from build123d import *

# Parameters (mm, degrees)
FRONT_SKETCH_R      = 1.905
BOSS_EXTRUDE1_DEPTH = 50.8
CUT_EXTRUDE1_DEPTH  = 45.72
CUT_EXTRUDE2_DEPTH  = 274.638700861
CUT_EXTRUDE3_DEPTH  = 18.03621965
SKETCH6_W           = 6.524310643
SKETCH6_H           = 22.300846009
SKETCH6_R           = 1.524
SKETCH6_W_2         = 6.962786951
BOSS_EXTRUDE2_DEPTH = 10.16


with BuildPart() as part:
    # front_sketch → Boss-Extrude1 (new body)
    with BuildSketch(Plane(origin=(0, 0, 0), x_dir=(1, 0, 0), z_dir=(0, 1, 0))):
        with BuildLine():
            Line((-94.961375831, 124.478458264), (-121.345326632, 110.234521439))
            ThreePointArc((-121.345326632, 110.234521439), (-122.32001306, 109.300728329), (-122.678671172, 107.99944144))
            Line((-122.678671172, 107.99944144), (-122.678671172, 48.810796684))
            Line((-122.678671172, 48.810796684), (-140.250849959, 48.810796684))
            Line((-140.250849959, 48.810796684), (-140.250849959, -56.645199257))
            Line((-140.250849959, -56.645199257), (-119.167015715, -56.645199257))
            Line((-119.167015715, -56.645199257), (-119.167015715, -126.112255785))
            Line((-119.167015715, -126.112255785), (-95.601645083, -136.460242597))
            Line((-95.601645083, -136.460242597), (-95.601645083, -142.810242597))
            Line((-95.601645083, -142.810242597), (-105.798207048, -142.810242597))
            ThreePointArc((-105.798207048, -142.810242597), (-119.167015715, -139.007347839), (-128.532661201, -128.737404395))
            ThreePointArc((-128.532661201, -128.737404395), (-157.286213724, -5.861503432), (-127.918775374, 116.869125935))
            ThreePointArc((-127.918775374, 116.869125935), (-118.556014486, 127.058910858), (-105.241228699, 130.828458264))
            Line((-105.241228699, 130.828458264), (-94.961375831, 130.828458264))
            Line((-94.961375831, 130.828458264), (-94.961375831, 124.478458264))
        make_face()
        with Locations((-131.296368682, 71.963600743)):
            Circle(FRONT_SKETCH_R, mode=Mode.SUBTRACT)
        with Locations((-131.296368682, -86.786399257)):
            Circle(FRONT_SKETCH_R, mode=Mode.SUBTRACT)
    extrude(amount=BOSS_EXTRUDE1_DEPTH)

    # Sketch1 → Cut-Extrude1 (cut)
    with BuildSketch(Plane(origin=(0, 50.8, 0), x_dir=(1, 0, 0), z_dir=(0, 1, 0))):
        Polygon((-122.678671172, 48.810796684), (-122.678671172, 107.99944144), (-138.833286115, 78.405119062), (-140.250849959, 48.810796684), align=None)
        Polygon((-119.167015715, -56.645199257), (-140.250849959, -56.645199257), (-139.542068037, -96.192486205), (-119.167015715, -126.112255785), align=None)
    extrude(amount=-CUT_EXTRUDE1_DEPTH, mode=Mode.SUBTRACT)

    # Sketch3 → Cut-Extrude2 (cut, through all)
    with BuildSketch(Plane.XY.offset(142.810242597)):
        Polygon((-94.961375831, 50.8), (-157.287069608, 21.270817167), (-157.287069608, 50.8), align=None)
    extrude(amount=-CUT_EXTRUDE2_DEPTH, mode=Mode.SUBTRACT)

    # Sketch4 → Cut-Extrude3 (cut, through all)
    with BuildSketch(Plane(origin=(-140.250849959, 0, 0), x_dir=(0, 0, -1), z_dir=(1, 0, 0))):
        Polygon((-24.404629664, 24.144542412), (20.256333242, 24.144542412), (20.256333242, 5.094542412), (20.256333242, 1.843696403), (-24.404629664, 1.843696403), (-24.404629664, 5.094542412), align=None)
    extrude(amount=-CUT_EXTRUDE3_DEPTH, mode=Mode.SUBTRACT)

    # Sketch6 → Boss-Extrude2 (add)
    with BuildSketch(Plane(origin=(-140.250849959, 0, 0), x_dir=(0, 0, -1), z_dir=(1, 0, 0))):
        with Locations((-21.142474343, 12.994119407)):
            Rectangle(SKETCH6_W, SKETCH6_H)
        with Locations((-20.530013168, 12.991512488)):
            Circle(SKETCH6_R, mode=Mode.SUBTRACT)
        with Locations((16.774939767, 12.994119407)):
            Rectangle(SKETCH6_W_2, SKETCH6_H)
        with Locations((16.553986832, 12.991512488)):
            Circle(SKETCH6_R, mode=Mode.SUBTRACT)
    extrude(amount=-BOSS_EXTRUDE2_DEPTH)


solid = part.part
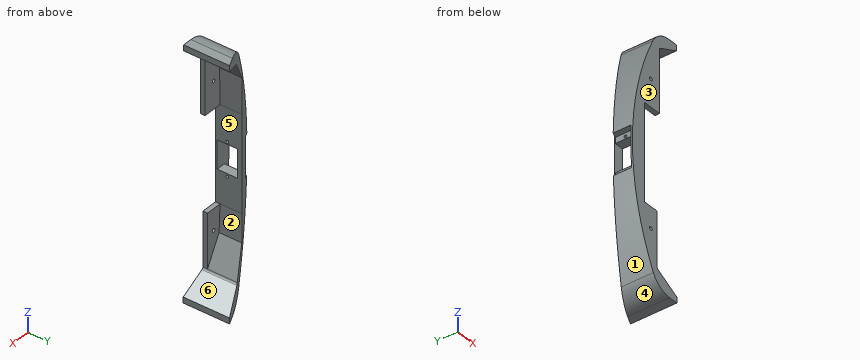
Geometry check sheet. Reference: the model listing, model coordinates, mm. Face numbers are marked on the shaded views. A direction names the side the tool comes from. Give positions to 0.01 mm unless a question says otherwise; leave off trailing zeros. Write each loop counter-clockwise with the first axis right and the second up, starting at its lowest first coordinate (ties: lowest second). Pieces come first, ordered by that corner, then holes.
1) Go/stop test with flat-tipped pins: pin 1 Ø3.5 at (x, z) = (-131.3, 86.79) entering from -Y; pin 2 Ø3.5 at (y, z) = (11.5, -16) entering from -X; pin 3 Ø9 at (x, z) = (-133, -89.5) entering from +Y; pin 4 Ø1.5 at (y, z) = (3, -71.5) entering from +X. Record where each tip stops, or that it passes through.
Values follow:
pin 1: passes through
pin 2: stops at x = -150.41
pin 3: stops at y = 33.88
pin 4: stops at x = -122.68
2) Set-up check for the marked faces 1 and 2: record each of +Z, -Z, +X, -X, +Y, -Y from which the full face is reachable in a straight line by a thin tool's end or side.
Values follow:
face 1: -X, +Y, -Y
face 2: +X, +Y
3) Release check for a two-part mould opening along Z. For the marked faces 3, 4, 5 and 6 record: released by +Z, released by -Z, zero draft, split by the parting line, or undercut.
Values follow:
face 3: zero draft
face 4: released by -Z
face 5: undercut
face 6: undercut
4) Cross-section at A-A (y = 8). Record the boundary of the cut face in (x, z), plus the area to 3 significant figures.
Values follow:
outline: (-156.7, 24.4) - (-150.41, 24.4) - (-150.41, 17.88) - (-140.25, 17.88) - (-140.25, 56.65) - (-139.54, 96.19) - (-119.17, 126.11) - (-95.6, 136.46) - (-95.6, 142.81) - (-105.8, 142.81) arc R25.4 ccw to (-128.53, 128.74) arc R274 ccw to start; (-155.97, -20.26) arc R274 ccw to (-127.92, -116.87) arc R25.4 ccw to (-105.24, -130.83) - (-94.96, -130.83) - (-94.96, -124.48) - (-121.35, -110.23) arc R2.54 cw to (-122.68, -108) - (-138.83, -78.41) - (-140.25, -48.81) - (-140.25, -13.29) - (-150.41, -13.29) - (-150.41, -20.26) - close
area: 2,780 mm2
5) Cross-section at D-D (x = -99.5). Record the boundary of the cut face in (y, z).
Values follow:
outline: (0, -130.83) - (48.65, -130.83) - (48.65, -122.03) - (0, -122.03) - close; (0, 134.75) - (48.65, 134.75) - (48.65, 142.81) - (0, 142.81) - close
6) Thickness scan on line 1 (X direction, y = 7.5, z = -19); line 2 (Z direction, x = -117.5, y = 26.5); line 3 (Y direction, x = -142, z = -12). Record the ranges inside material, lowest first.
Values follow:
line 1: x = -150.41 to -140.25
line 2: z = -127.67 to -112.31, 126.84 to 139.95
line 3: y = 0 to 1.84, 24.14 to 28.51
7) Cross-section at C-C (z = 13). Record the boundary of the cut face in (x, y).
Values follow:
outline: (-157.21, 0) - (-140.25, 0) - (-140.25, 1.84) - (-157.21, 1.84) - close; (-151.22, 24.14) - (-140.25, 24.14) - (-140.25, 29.34) - close
8) Cross-section at B-B (x = -145.5). Record the boundary of the cut face in (y, z).
Values follow:
outline: (0, -72.95) - (26.86, -72.95) - (26.86, 86.05) - (0, 86.05) - close; hole (1.84, -13.29) - (24.14, -13.29) - (24.14, 17.88) - (1.84, 17.88) - close; hole circle Ø3.05 at (12.99, -16.55); hole circle Ø3.05 at (12.99, 20.53)
